Answer from the drawing. Dimensions are ordinates in mm from the lowest x, y and z of the part. Give positions to 0.01 mm unless a question says otherwise; leave off trailing zeros. Write each loop counter-clockwise with the first axis right and the second up, starting at its lowest first coordinate (ties: lowest second). Pieces come first, ordered by that corner, then holes. Notation, with made-up numbers: (-29, 67) - (-10, 67) arc R27 ccw to (-10, 103) - close; hole circle Ø8 at (-30, 85.5). An arc over 180 degrees is marked (long way). Write item = value, one per line.
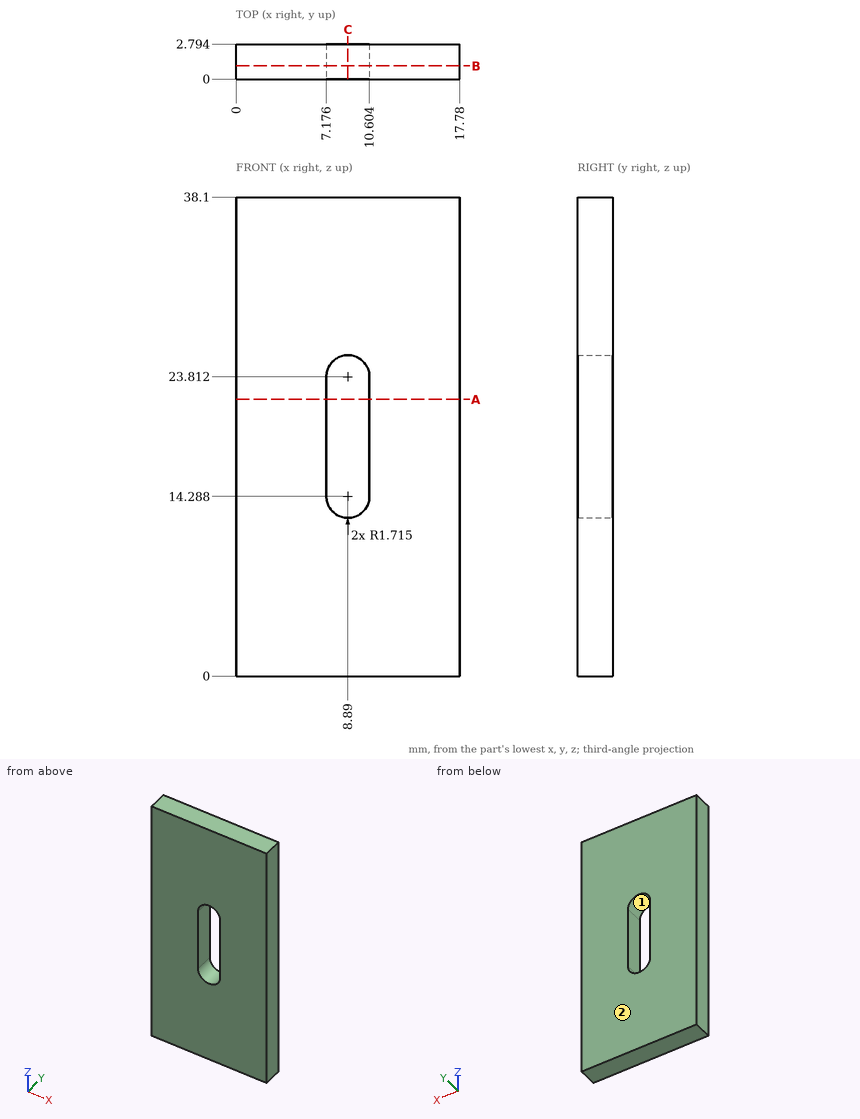
1. For a pull along X with two mould halves and no side action, classify the marked faces 1 and 2 as pulls with the +X half, pulls with the -X half, needs draft (parallel to the pull), parting line crosses it, or undercut.
Solution:
face_1 = undercut
face_2 = needs draft
2. Find section B-B, the plane y = 1.05. Give the vertices of the cut face in (x, z) (1 decimal).
Solution:
outline = (0, 0) - (17.8, 0) - (17.8, 38.1) - (0, 38.1) - close; hole (7.2, 14.3) arc R1.7 ccw to (10.6, 14.3) - (10.6, 23.8) arc R1.7 ccw to (7.2, 23.8) - close
3. Straight lines are drawn through the part: line 1 (X direction, y = 0.4, z = 21.5) (1 decimal); line 2 (Z direction, x = 9, y = 1.8); line 3 (Z direction, x = 7.5, y = 0.6) (1 decimal). For each, find the intervals that lie inside material, in ascending order.
Solution:
line_1 = 0 to 7.2, 10.6 to 17.8
line_2 = 0 to 12.58, 25.52 to 38.1
line_3 = 0 to 13.3, 24.8 to 38.1
4. Find section C-C, the plane x = 8.89. Give the vertices of the cut face in (y, z) (1 decimal).
Solution:
outline = (0, 0) - (2.8, 0) - (2.8, 12.6) - (0, 12.6) - close; (0, 25.5) - (2.8, 25.5) - (2.8, 38.1) - (0, 38.1) - close
5. Find section A-A, the plane z = 22. Give the vertices of the cut face in (x, y) (1 decimal).
Solution:
outline = (0, 0) - (7.2, 0) - (7.2, 2.8) - (0, 2.8) - close; (10.6, 0) - (17.8, 0) - (17.8, 2.8) - (10.6, 2.8) - close
